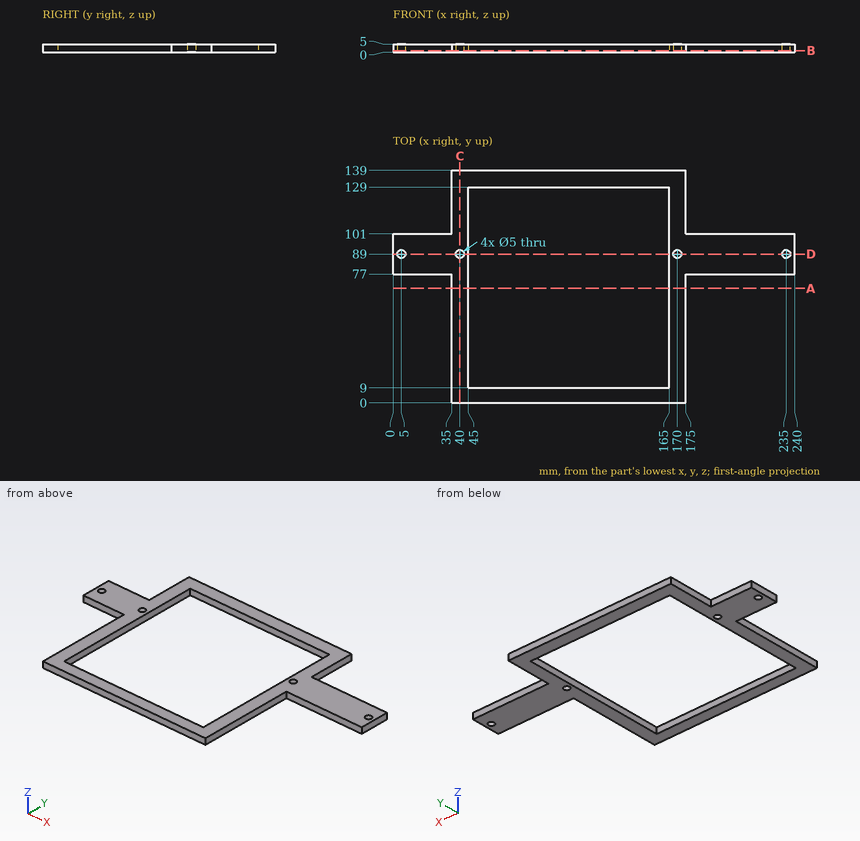
The drawing under review shows one solid part. Ordinate dimensions are in mm from its lowest x, y, z. Round coordinates to 2 decimals unless told otherwise and drop trailing zeros. Write each loop counter-clockwise with the first axis right and the second up, starting at its lowest first coordinate (ties: lowest second). Pieces come first, ordered by that corner, then holes. Notation, with made-up numbers: (44, 69) - (60, 69) arc R32 cw to (60, 95) - close; hole circle Ø6 at (26, 43.25). An arc over 180 degrees is marked (long way). Write each question's results on one line, items separated by ' | '.
Item 1: Take a section at D-D on y = 89. State the section outline as (x, z) points.
Calculated:
outline: (0, 0) - (2.5, 0) - (2.5, 5) - (0, 5) - close; (7.5, 0) - (37.5, 0) - (37.5, 5) - (7.5, 5) - close; (42.5, 0) - (45, 0) - (45, 5) - (42.5, 5) - close; (165, 0) - (167.5, 0) - (167.5, 5) - (165, 5) - close; (172.5, 0) - (232.5, 0) - (232.5, 5) - (172.5, 5) - close; (237.5, 0) - (240, 0) - (240, 5) - (237.5, 5) - close
Item 2: For pin 1 (6 mm diameter, centred on x = 40, y = 89, fed in from +Z); pin 2 (1.5 mm diameter, centred on y = 112.5, z = 3, fed in from +X); pin 3 (1.5 mm diameter, centred on y = 52, z = 2, fed in from -X); pin 4 (1.5 mm diameter, centred on x = 207, z = 0.5, fed in from -Y), all flat-tipped, find the tip position at first contact; note any pin that passes through.
Calculated:
pin 1: stops at z = 5 | pin 2: stops at x = 175 | pin 3: stops at x = 35 | pin 4: stops at y = 77
Item 3: To check wall thickness, follow line 1 along X through (y, z) = (89, 1.75); line 2 along Y through (x, z) = (5, 3.05); line 3 along Y through (x, z) = (164, 3.3). State the ranges of each line that lie inside material, in increasing order. Write a range as from..to.
Calculated:
line 1: x = 0..2.5, 7.5..37.5, 42.5..45, 165..167.5, 172.5..232.5, 237.5..240 | line 2: y = 77..86.5, 91.5..101 | line 3: y = 0..9, 129..139
Item 4: Take a section at B-B on z = 1. State the section outline as (x, y) points.
Calculated:
outline: (0, 77) - (35, 77) - (35, 0) - (175, 0) - (175, 77) - (240, 77) - (240, 101) - (175, 101) - (175, 139) - (35, 139) - (35, 101) - (0, 101) - close; hole circle Ø5 at (5, 89); hole circle Ø5 at (40, 89); hole (45, 9) - (165, 9) - (165, 129) - (45, 129) - close; hole circle Ø5 at (170, 89); hole circle Ø5 at (235, 89)
Item 5: Take a section at C-C on x = 40. State the section outline as (y, z) points.
Calculated:
outline: (0, 0) - (86.5, 0) - (86.5, 5) - (0, 5) - close; (91.5, 0) - (139, 0) - (139, 5) - (91.5, 5) - close
Item 6: Take a section at A-A on y = 68.5. State the section outline as (x, z) points.
Calculated:
outline: (35, 0) - (45, 0) - (45, 5) - (35, 5) - close; (165, 0) - (175, 0) - (175, 5) - (165, 5) - close
